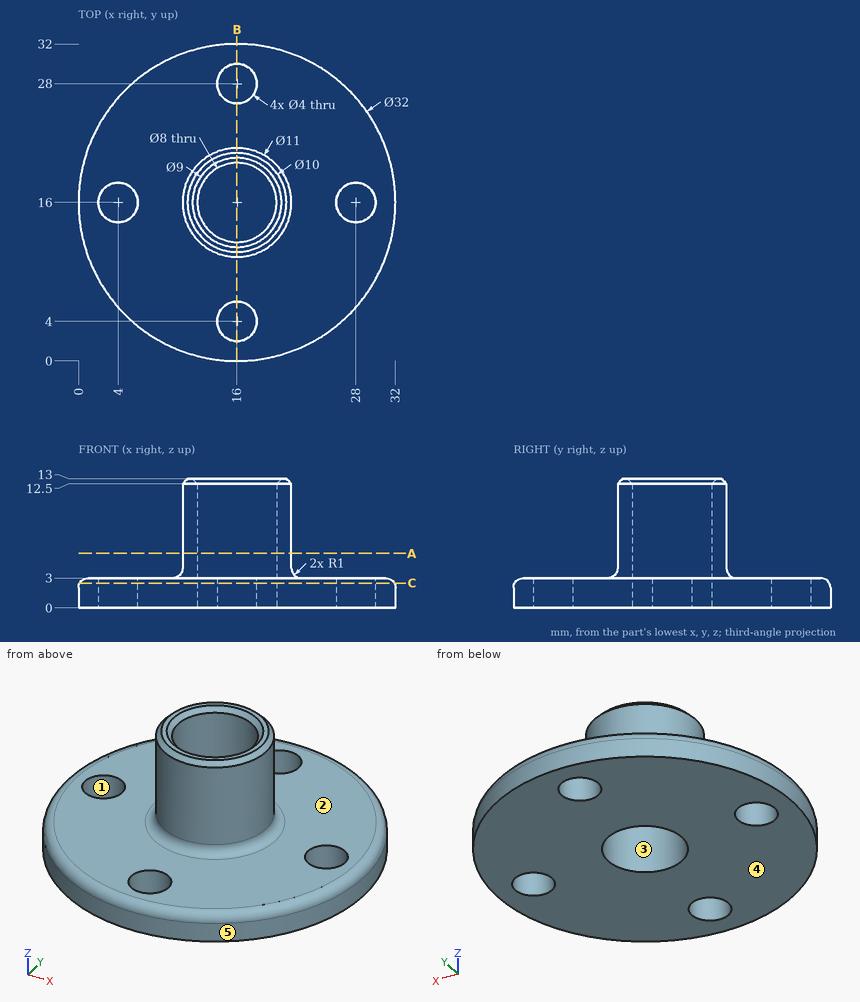
The figure shows three views and two pictorial views of one solid part (mm, origin at its lowest corner). Answer the questions. A direction names the side the tool comes from. Coordinates: 2 decimals unless noted, no trailing zeros. Loops run counter-clockwise (first coordinate to the right, second up) from the corner with the lowest first, then second, coordinate; pieces in that order, holes last. Notation, with made-up numbers: (-6.75, 4) - (45.25, 4) arc R34 cw to (45.25, 42) - close; hole circle Ø5 at (-17.5, -14). An arc over 180 degrees is marked (long way). Answer in a Markdown table with one row per item.
Q1. Straight lines are drawn through the part: line 1 along Y through (x, z) = (16, 6.25); line 2 along X through (y, z) = (14.5, 1); line 3 along Z through (x, y) = (22, 4). For each, find the intervals that lie inside material, in ascending order. Write a range as [from, to].
Here are the results:
| item | result |
|---|---|
| line 1 | y = [10.5, 12], [20, 21.5] |
| line 2 | x = [0.07, 2.68], [5.32, 12.29], [19.71, 26.68], [29.32, 31.93] |
| line 3 | z = [0, 3] |
Q2. Find section C-C on z = 2.5. Write down the section's boundary in (x, y), plus the area to 3 significant figures.
Here are the results:
| item | result |
|---|---|
| outline | circle Ø31.73 at (16, 16); hole circle Ø4 at (4, 16); hole circle Ø8 at (16, 16); hole circle Ø4 at (16, 4); hole circle Ø4 at (16, 28); hole circle Ø4 at (28, 16) |
| area | 690 mm^2 |
Q3. For the marked faces 1 and 2, determine the directions among +Z, -Z, +X, -X, +Y, -Y from which every point of the face is accessible in a straight line to the end or side of a thin tool.
Here are the results:
| item | result |
|---|---|
| face 1 | +Z, -Z |
| face 2 | +Z |
Q4. The mould has two halves that part along Y. Classify the marked faces 3, 4 and 5: pulls with the +Y half, pulls with the -Y half, needs draft (parallel to the pull), parting line crosses it, or undercut.
Here are the results:
| item | result |
|---|---|
| face 3 | undercut |
| face 4 | needs draft |
| face 5 | parting line crosses it |
Q5. Find section A-A on z = 5.5. Write down the section's boundary in (x, y), plus the area to 3 significant figures.
Here are the results:
| item | result |
|---|---|
| outline | circle Ø11 at (16, 16); hole circle Ø8 at (16, 16) |
| area | 44.8 mm^2 |
Q6. Given P1, Ø6.5, axis at x = 16, y = 16, coming from the -Z side; P2, Ø4, axis at x = 7, y = 14.5, coming from the +Z side; P3, Ø6, axis at y = 8, z = 3, coming from the -X side; P4, Ø2, axis at y = 28.5, z = 3.5, coming from the -X side, each flat-ended and moving along its own axis, determine where each tip first touches the part or whether it passes through.
Here are the results:
| item | result |
|---|---|
| P1 | passes through |
| P2 | stops at z = 3 |
| P3 | stops at x = 0.85 |
| P4 | stops at x = 5.74 |
Q7. Find section B-B on x = 16. Count the separate pieces of the cut face and the enclosed holes in it, plus the area to 3 significant figures.
Here are the results:
| item | result |
|---|---|
| separate pieces | 4 |
| enclosed holes | 0 |
| area | 77.5 mm^2 |
